The listing builds one solid part. Answer for the finished solid, in the listing's coordinates (mm). A direction names the side the tool comes from. Round coordinates to 2 decimals unless told otherwise and drop trailing zeros. Order: outer loops, then holes, each group sorted by start corner. A loop starts at its lowest first (then second) coordinate and runs counter-clockwise, first axis right, second up. Notation, with made-up numbers: (35, -19) - (86, -19) arc R12 cw to (86, -8) - close; hole circle Ø8 at (-23, -10.75). An arc over 180 degrees is marked (long way). One line per item, written item: value. Start each with the question number.
1. Section A-A, the plane z = 1.15 is taken. Give the vertices of the cut face in (x, y).
2. For a pull along X with two mould halves and no side action, classify faces 6 (the flat face through (5, 44.448, 3)), 7 (the flat face through (4.58, 4.49, 0.99)), 8 (the cylindrical face through (8.54, 12.71, 3.48)) as released by +X, released by -X, zero draft, split by the parting line, or undercut.
3. Section C-C, the plane y = 33.5 is taken. Give the vertices of the cut face in (x, z), then the cut area to 3 significant figures.
4. A tool of negligible diameter and unlimited length cuts with its end or side. For faces 1 (the flat face through (75, 44.448, 3)), 2 (the flat face through (5, 14.57, 3)), 3 (the flat face through (67.674, 11, 3)), 4 (the flat face through (75, 41.948, 3)), 5 (the flat face through (5, 44.702, 1)), from which of +Z, -Z, +X, -X, +Y, -Y can it reach the whole face along a straight path? Write none if from no direction.
5. Section D-D, the plane x = 36 is taken. Give the vertices of the cut face in (y, z), then the cut area to 3 significant figures.
6. Flat-ended cylindrical pins translate along their axes: P1, Ø4, axis at x = 68.5, y = 26.5, coming from the +Z side; P2, Ø0.8, axis at x = 17.5, z = 3.5, coming from the +Y side; P3, Ø1, axis at x = 6.5, z = 0.5, coming from the -Y side. Find the tip coordinate at first contact, or state that the pin passes through.
7. Straight lines are drawn through the part: line 1 (Y direction, x = 13.5, z = 2.75); line 2 (X direction, y = 28.5, z = 1.6); line 3 (X direction, y = 23, z = 2.25). For each, find the intervals that lie inside material, in ascending order.
8. Section B-B, the plane y = 13.32 is taken. Give the vertices of the cut face in (x, z), then the cut area to 3 significant figures.
from build123d import *

# Parameters (mm, degrees)
BOSS_EXTRUDE3_DEPTH = 2
SKETCH7_R           = 1
SKETCH7_W           = 2.5
SKETCH7_H           = 2.5
BOSS_EXTRUDE5_DEPTH = 3
SKETCH15_R          = 6.016109345
SKETCH15_R_2        = 2.966709341
CUT_EXTRUDE5_DEPTH  = 3
CUT_EXTRUDE6_DEPTH  = 3
CUT_EXTRUDE7_DEPTH  = 10
SKETCH30_W          = 2
SKETCH30_H          = 65
BOSS_EXTRUDE6_DEPTH = 5
SKETCH31_R          = 3.139995771
SKETCH31_R_2        = 5.842822915
CUT_EXTRUDE8_DEPTH  = 5
SKETCH33_W          = 2.81704287
SKETCH33_H          = 5.093792668
CUT_EXTRUDE9_DEPTH  = 5


with BuildPart() as part:
    # Sketch2 → Boss-Extrude3 (new body)
    with BuildSketch(Plane.XY):
        Polygon((62.078732257, 67), (7.070378023, 67), (2.153513577, 62.087886246), (2.153513577, 6.916864445), (7.070378023, 2), (62.078732257, 2), (67.153513577, 7.083274694), (67.153513577, 61.921636784), align=None)
        with BuildLine():
            ThreePointArc((12.561398281, 29.386897281), (12.405099811, 29.087669445), (12.28230409, 28.773205265))
            ThreePointArc((12.28230409, 28.773205265), (9.332354964, 25.48092154), (6.384978263, 28.775508397))
            ThreePointArc((6.384978263, 28.775508397), (6.272687262, 29.080787813), (6.128559615, 29.372390302))
            ThreePointArc((6.128559615, 29.372390302), (9.319946418, 40.479834047), (12.561398281, 29.386897281))
        make_face(mode=Mode.SUBTRACT)
        with BuildLine():
            Line((7.315683042, 44.45), (3.053513577, 44.45))
            Line((3.053513577, 44.45), (3.053513577, 49.55))
            Line((3.053513577, 49.55), (15.603513577, 49.55))
            Line((15.603513577, 49.55), (15.603513577, 44.45))
            Line((15.603513577, 44.45), (11.175073004, 44.45))
            ThreePointArc((11.175073004, 44.45), (9.245378023, 45.49849), (7.315683042, 44.45))
        make_face(mode=Mode.SUBTRACT)
    boss_extrude3 = extrude(amount=BOSS_EXTRUDE3_DEPTH)

    # Sketch7 → Boss-Extrude5 (add)
    with BuildSketch(Plane.XY.offset(2)):
        with BuildLine():
            Line((15.753513577, 14.57), (11.264187035, 14.57))
            ThreePointArc((11.264187035, 14.57), (9.333513577, 15.62), (7.40284012, 14.57))
            Line((7.40284012, 14.57), (2.153513577, 14.57))
            Line((2.153513577, 14.57), (2.153513577, 12.07))
            Line((2.153513577, 12.07), (7.033513577, 12.07))
            Line((7.033513577, 12.07), (7.40284012, 12.07))
            ThreePointArc((7.40284012, 12.07), (9.333513577, 11.02), (11.264187035, 12.07))
            Line((11.264187035, 12.07), (11.633513577, 12.07))
            Line((11.633513577, 12.07), (15.753513577, 12.07))
            Line((15.753513577, 12.07), (15.753513577, 14.57))
        make_face()
        with Locations((9.333513577, 13.32)):
            Circle(SKETCH7_R, mode=Mode.SUBTRACT)
        with BuildLine():
            Line((11.633513577, 9.547776159), (11.633513577, 12.07))
            Line((11.633513577, 12.07), (11.264187035, 12.07))
            ThreePointArc((11.264187035, 12.07), (9.333513577, 11.02), (7.40284012, 12.07))
            Line((7.40284012, 12.07), (7.033513577, 12.07))
            Line((7.033513577, 12.07), (7.033513577, 9.547776159))
            Line((7.033513577, 9.547776159), (11.633513577, 9.547776159))
        make_face()
        with Locations((17.003513577, 13.32)):
            Rectangle(SKETCH7_W, SKETCH7_H)
        with BuildLine():
            Line((15.753513577, 16.534568208), (15.753513577, 14.57))
            Line((15.753513577, 14.57), (18.253513577, 14.57))
            Line((18.253513577, 14.57), (18.253513577, 16.534568208))
            Line((18.253513577, 16.534568208), (18.253513577, 44.45))
            Line((18.253513577, 44.45), (15.753513577, 44.45))
            Line((15.753513577, 44.45), (15.753513577, 44.44849))
            Line((15.753513577, 44.44849), (11.17605148, 44.44849))
            ThreePointArc((11.17605148, 44.44849), (11.17556239, 44.449245096), (11.175073004, 44.45))
            ThreePointArc((11.175073004, 44.45), (10.343450652, 45.219439406), (9.245378023, 45.49849))
            ThreePointArc((9.245378023, 45.49849), (8.147305393, 45.219439406), (7.315683042, 44.45))
            ThreePointArc((7.315683042, 44.45), (7.315193656, 44.449245096), (7.314704565, 44.44849))
            Line((7.314704565, 44.44849), (2.153513577, 44.44849))
            Line((2.153513577, 44.44849), (2.153513577, 41.94849))
            Line((2.153513577, 41.94849), (7.314704565, 41.94849))
            ThreePointArc((7.314704565, 41.94849), (9.245378023, 40.89849), (11.17605148, 41.94849))
            Line((11.17605148, 41.94849), (15.753513577, 41.94849))
            Line((15.753513577, 41.94849), (15.753513577, 16.534568208))
        make_face()
        with Locations((9.245378023, 43.19849)):
            Circle(SKETCH7_R, mode=Mode.SUBTRACT)
    boss_extrude5 = extrude(amount=BOSS_EXTRUDE5_DEPTH)

    # Mirror4: Boss-Extrude3, Boss-Extrude5 across plane
    add(boss_extrude3.mirror(Plane.ZY.offset(-34.653513577)))
    add(boss_extrude5.mirror(Plane.ZY.offset(-34.653513577)))

    # Sketch15 → Cut-Extrude5 (cut)
    with BuildSketch(Plane.XY.offset(2)):
        with Locations((9.333513577, 34.46374)):
            Circle(SKETCH15_R)
        with Locations((9.333513577, 28.447630655)):
            Circle(SKETCH15_R_2)
    cut_extrude5 = extrude(amount=-CUT_EXTRUDE5_DEPTH, mode=Mode.SUBTRACT)

    # Sketch21 → Cut-Extrude6 (cut)
    with BuildSketch(Plane.XY.offset(2)):
        with BuildLine():
            Line((3.317404233, 44.701735967), (7.504616246, 44.701735967))
            ThreePointArc((7.504616246, 44.701735967), (9.245378023, 45.49849), (10.986139799, 44.701735967))
            Line((10.986139799, 44.701735967), (15.349622922, 44.701735967))
            Line((15.349622922, 44.701735967), (15.349622922, 49.701735967))
            Line((15.349622922, 49.701735967), (3.317404233, 49.701735967))
            Line((3.317404233, 49.701735967), (3.317404233, 44.701735967))
        make_face()
    extrude(amount=-CUT_EXTRUDE6_DEPTH, mode=Mode.SUBTRACT)

    # Sketch29 → Cut-Extrude7 (cut)
    with BuildSketch(Plane.XY.offset(2)):
        with BuildLine():
            Line((3.317404233, 44.795528635), (7.590244313, 44.795528635))
            ThreePointArc((7.590244313, 44.795528635), (9.245378023, 45.49849), (10.900511733, 44.795528635))
            Line((10.900511733, 44.795528635), (15.349622922, 44.795528635))
            Line((15.349622922, 44.795528635), (15.349622922, 49.795528635))
            Line((15.349622922, 49.795528635), (3.317404233, 49.795528635))
            Line((3.317404233, 49.795528635), (3.317404233, 44.795528635))
        make_face()
    cut_extrude7 = extrude(amount=-CUT_EXTRUDE7_DEPTH, mode=Mode.SUBTRACT)

    # Mirror9: Cut-Extrude7 across plane
    add(cut_extrude7.mirror(Plane.ZY.offset(-34.653513577)), mode=Mode.SUBTRACT)

    # Mirror5: Cut-Extrude5 across plane
    add(cut_extrude5.mirror(Plane.ZY.offset(-34.653513577)), mode=Mode.SUBTRACT)

    # SurfaceCut1
    split(bisect_by=Plane.ZY.offset(-34.653513577), keep=Keep.TOP)

    # Sketch30 → Boss-Extrude6 (add)
    with BuildSketch(Plane(origin=(34.653513577, 0, 0), x_dir=(0, 0, -1), z_dir=(1, 0, 0))):
        with Locations((-1, 34.5)):
            Rectangle(SKETCH30_W, SKETCH30_H)
    extrude(amount=BOSS_EXTRUDE6_DEPTH)

    # Mirror12: Boss-Extrude3, Boss-Extrude5 across plane
    add(boss_extrude3.mirror(Plane(origin=(39.653513577, 0, 0), x_dir=(0, 0, 1), z_dir=(1, 0, 0))))
    add(boss_extrude5.mirror(Plane(origin=(39.653513577, 0, 0), x_dir=(0, 0, 1), z_dir=(1, 0, 0))))

    # Sketch31 → Cut-Extrude8 (cut)
    with BuildSketch(Plane.XY.offset(2)):
        with Locations((9.333513577, 28.620917085)):
            Circle(SKETCH31_R)
        with Locations((9.333513577, 34.46374)):
            Circle(SKETCH31_R_2)
    extrude(amount=-CUT_EXTRUDE8_DEPTH, mode=Mode.SUBTRACT)

    # Sketch33 → Cut-Extrude9 (cut)
    with BuildSketch(Plane.XY.offset(2)):
        with Locations((13.562035012, 47.248632301)):
            Rectangle(SKETCH33_W, SKETCH33_H)
    extrude(amount=-CUT_EXTRUDE9_DEPTH, mode=Mode.SUBTRACT)


solid = part.part
Answer list:
1. outline: (2.15, 6.92) - (7.07, 2) - (72.24, 2) - (77.15, 6.92) - (77.15, 62.09) - (72.24, 67) - (7.07, 67) - (2.15, 62.09) - close; hole (3.32, 44.7) - (7.5, 44.7) arc R2.3 cw to (10.99, 44.7) - (14.97, 44.7) - (14.97, 49.8) - (3.32, 49.8) - close; hole (6.27, 29.29) arc R3.14 ccw (long way) to (12.36, 29.46) arc R5.84 ccw to (12.15, 39.58) - (12.15, 39.78) arc R6.02 ccw to start; hole (63.7, 44.45) - (68.13, 44.45) arc R2.3 cw to (71.99, 44.45) - (76.25, 44.45) - (76.25, 49.55) - (63.7, 49.55) - close; hole (66.75, 29.39) arc R3.1 cw to (67.02, 28.77) arc R2.97 ccw (long way) to (72.92, 28.78) arc R3.05 cw to (73.18, 29.37) arc R6.02 ccw (long way) to start
2. face 6: zero draft
2. face 7: released by -X
2. face 8: undercut
3. outline: (2.15, 0) - (3.4, 0) - (3.4, 2) - (2.15, 2) - close; (15.1, 0) - (64.04, 0) - (64.04, 2) - (63.55, 2) - (63.55, 5) - (61.05, 5) - (61.05, 2) - (18.25, 2) - (18.25, 5) - (15.75, 5) - (15.75, 2) - (15.1, 2) - close; (75.91, 0) - (77.15, 0) - (77.15, 2) - (75.91, 2) - close
3. area: 118 mm²
4. face 1: +Z, +X, +Y
4. face 2: +Z, -X
4. face 3: +Z, -Y
4. face 4: +Z, +X
4. face 5: +Z, -Z
5. outline: (2, 0) - (67, 0) - (67, 2) - (2, 2) - close
5. area: 130 mm²
6. P1: stops at z = 2
6. P2: stops at y = 44.45
6. P3: stops at y = 2.07
7. line 1: y = 12.07 to 14.57, 41.95 to 44.45
7. line 2: x = 2.15 to 6.2, 12.47 to 67.01, 72.94 to 77.15
7. line 3: x = 15.75 to 18.25, 61.05 to 63.55
8. outline: (2.15, 0) - (77.15, 0) - (77.15, 5) - (70.97, 5) - (70.97, 2) - (68.97, 2) - (68.97, 5) - (61.05, 5) - (61.05, 2) - (18.25, 2) - (18.25, 5) - (10.33, 5) - (10.33, 2) - (8.33, 2) - (8.33, 5) - (2.15, 5) - close
8. area: 235 mm²
